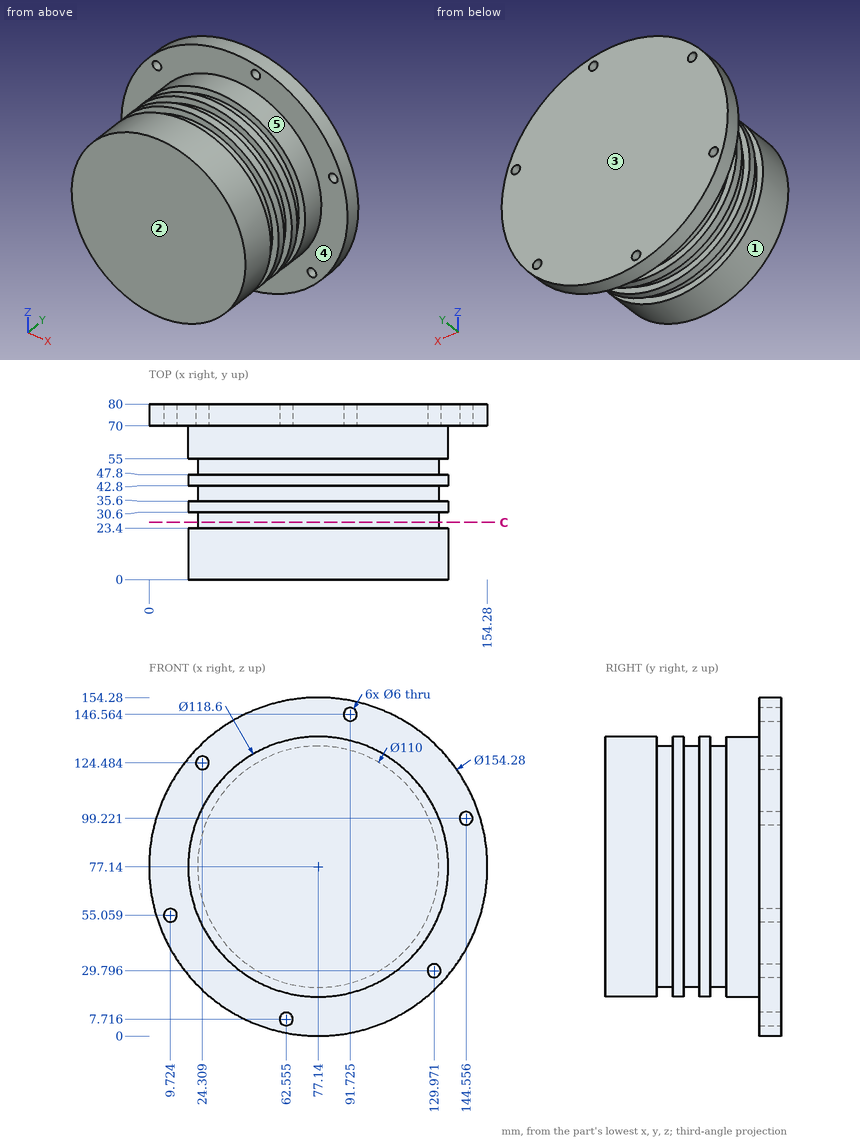
Job drawing, mm, ordinate dimensions from the low corner. One solid piece. A direction names the side the tool comes from. Give positions to 0.01 mm unless a question says otherwise; leave off trailing zeros. Write each loop counter-clockwise with the first axis right and the second up, starting at its lowest first coordinate (ties: lowest second). Pieces come first, ordered by that corner, then holes. Notation, with made-up numbers: (-23, 69.5) -> (-5, 69.5) arc R21 ccw to (-5, 105.5) -> close; hole circle Ø2 at (50.25, 58.25). An arc over 180 degrees is marked (long way). Return JSON: item names as keys, results as strings.
Item 1: Two-plate mould, pull along Y, no slides. Class the marked faces 3, 4 and 5: +Y half, -Y half, draft (parallel to the pull), parting line (faces both ways), or undercut.
Answer below:
{"face 3": "+Y half", "face 4": "-Y half", "face 5": "draft"}
Item 2: Tool access for the marked faces 1 and 2: list every direction of +Z, -Z, +X, -X, +Y, -Y with a clear straight run to the whole face (end or side of a thin tool).
Answer below:
{"face 1": "-Y", "face 2": "+Z, -Z, +X, -X, -Y"}
Item 3: Band-saw the part on C-C (y = 26). List the corners of the cut face in (x, z), then the cut area to 3 significant figures.
Answer below:
{"outline": "circle Ø110 at (77.14, 77.14)", "area": "9,500 mm2"}
Item 4: Drop flat-ended pins along their axis: pin 1 (12 mm diameter, centred on x = 112.5, y = 35, fed in from +Z); pin 2 (10 mm diameter, centred on y = 43, z = 64, fed in from -X); pin 3 (2 mm diameter, centred on y = 18, z = 69, fed in from +X). Give the stop position or say it passes through.
Answer below:
{"pin 1": "stops at z = 128.66", "pin 2": "stops at x = 18.4", "pin 3": "stops at x = 136.01"}
Item 5: Drill centre lines: probe 1 along Y at (x, z) = (36, 18.5); probe 2 along X at (y, z) = (27, 66.5); probe 3 along X at (y, z) = (15, 48.5) (1 decimal). Where is each one in solid material? Low to high.
Answer below:
{"probe 1": "y = 70 to 80", "probe 2": "x = 23.18 to 131.1", "probe 3": "x = 25.2 to 129.1"}
